Source: three-view drawing plus pictorial views. Frame: mm from the lowest corner of the part. A direction names the side the tool comes from. Give positions to 0.01 mm unless a question says otherwise; leave off trailing zeros. Order: outer loops, then holes, each group sorted by start corner. A loop starts at its lowest first (then second) coordinate and runs counter-clockwise, first axis right, second up. Notation, with made-up numbers: M -17,-19 L -11,-19 A28 cw -11,12 Z; hole C -7.75,50.25 d5. An arc over 180 degrees is marked long. Use CSV: the item, a comma, the result in double quotes.
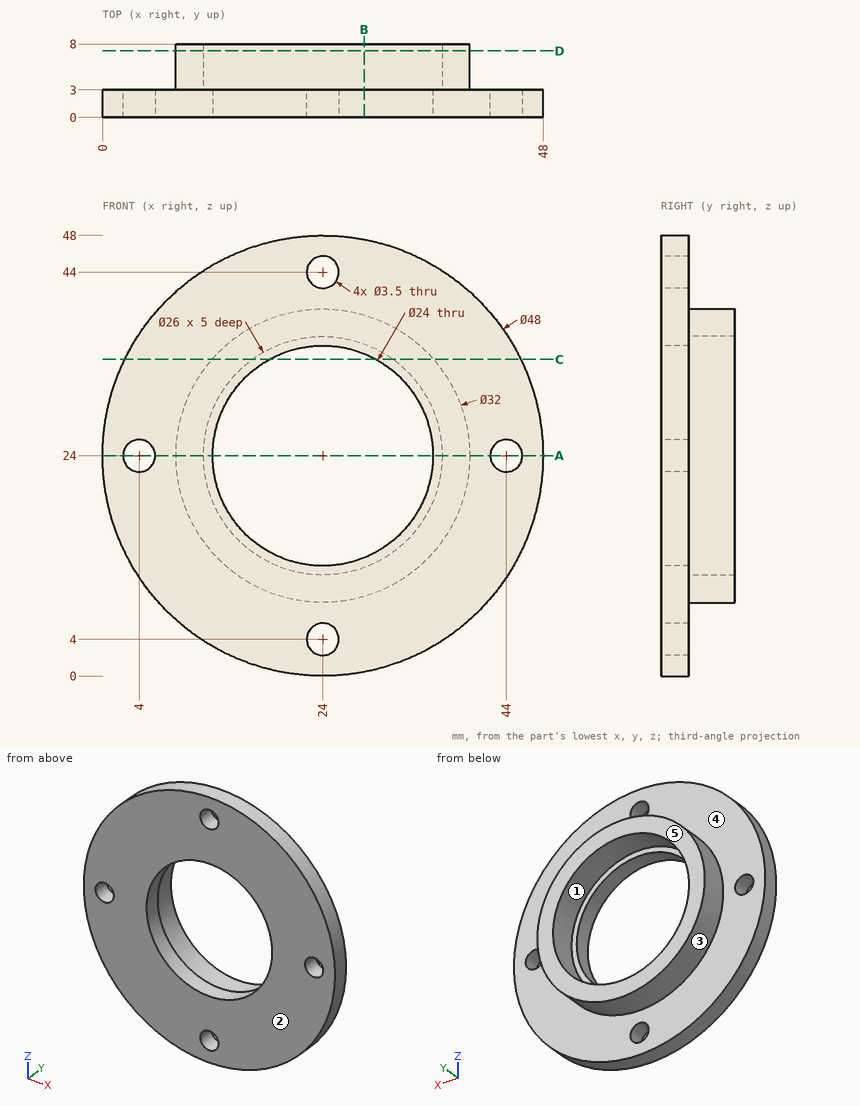
1. Section A-A, the plane z = 24. Return the cut outline in (x, y).
Answer:
outline,"M 0,0 L 2.25,0 L 2.25,3 L 0,3 Z; M 5.75,0 L 12,0 L 12,3 L 11,3 L 11,8 L 8,8 L 8,3 L 5.75,3 Z; M 36,0 L 42.25,0 L 42.25,3 L 40,3 L 40,8 L 37,8 L 37,3 L 36,3 Z; M 45.75,0 L 48,0 L 48,3 L 45.75,3 Z"
2. Reachability of the marked faces 4 and 5 from +Z, -Z, +X, -X, +Y, -Y: full face, straight path, thin tool, end or side. Return the list, or none.
Answer:
face 4,"+Y"
face 5,"+Z, -Z, +X, -X, +Y"
3. Pull-direction query (X, two-part tool) for the marked faces 1, 2 and 3; classes: +X half, -X half, draft (parallel to the pull), parting line (faces both ways), or undercut.
Answer:
face 1,"undercut"
face 2,"draft"
face 3,"parting line"
4. Pin query (flat end, axial travel): pin 1 Ø12 at (x, z) = (11, 7.5) entering from -Y; pin 2 Ø3 at (x, z) = (9, 43) entering from +Y; pin 3 Ø3 at (x, y) = (17, 5) entering from -Z (3 decimals). Return the tip coordinate at first contact, or that it passes through.
Answer:
pin 1,"y = 0"
pin 2,"y = 3"
pin 3,"z = 8.975"
5. Section B-B, the plane x = 28.5. Return the cut outline in (y, z), plus the area to 3 significant figures.
Answer:
outline,"M 0,0.43 L 3,0.43 L 3,8.65 L 8,8.65 L 8,11.8 L 3,11.8 L 3,12.88 L 0,12.88 Z; M 0,35.12 L 3,35.12 L 3,36.2 L 8,36.2 L 8,39.35 L 3,39.35 L 3,47.57 L 0,47.57 Z"
area,"106 mm2"
6. Line query: line 1 (Z direction, x = 24, y = 1.05); line 2 (X direction, y = 4, z = 33.5); line 3 (Y direction, x = 13, z = 45). Output: solid intervals per line, ascending.
Answer:
line 1,"0 to 2.25, 5.75 to 12, 36 to 42.25, 45.75 to 48"
line 2,"11.13 to 15.13, 32.87 to 36.87"
line 3,"0 to 3"
7. Section C-C, the plane z = 34.5. Return the cut outline in (x, y), plus the area to 3 significant figures.
Answer:
outline,"M 2.42,0 L 18.19,0 L 18.19,3 L 16.34,3 L 16.34,8 L 11.93,8 L 11.93,3 L 2.42,3 Z; M 29.81,0 L 45.58,0 L 45.58,3 L 36.07,3 L 36.07,8 L 31.66,8 L 31.66,3 L 29.81,3 Z"
area,"139 mm2"
8. Section D-D, the plane y = 7.25. Return the cut outline in (x, z), plus the area to 3 significant figures.
Answer:
outline,"C 24,24 d32; hole C 24,24 d26"
area,"273 mm2"
